Can you work these out from the drawing? Everything is in mm from the part's minimum corner. A direction names the side the tool comes from. Coordinates: 2 decimals unless noted, no trailing zeros. Loops run counter-clockwise (first coordinate to the right, second up) from the corner with the lowest first, then second, coordinate; pieces in that order, holes last. Notation, with made-up numbers: (-22.75, -15) -> (-10.75, -15) arc R24 cw to (-10.75, 22) -> close; hole circle Ø11 at (-4, -19.5). An arc over 180 degrees is marked (long way). Use one line per item in the form item = value. Start each with the question number.
(1) On a 3-axis mill with a long thin cutter (end or side, diameter ignored), from which of +Z, -Z, +X, -X, +Y, -Y can I reach the whole of each face in a straight line? I mean the marked faces 1, 2 and 3. Say none if no direction works.
(2) Thinking about a two-plate mould opening in X: for the marked faces 4, 5, 6 and 7, which applies, released by +X, released by -X, zero draft, split by the parting line, or undercut?
(3) I need wall thicknesses on line 1 (Y direction, x = 1, z = 12.75). Which ranges of the line are inside material? Lowest first, please. Write a range as [from, to].
(4) Imagine slicing it at A-A (x = 6.5). List the corners of the cut face in (y, z) for me, plus the area to 3 significant figures.
(5) I'm going to push a flat-ended pin straight in: pin 1 (0.6 mm diameter, centred on x = 7.5, y = 14, fed in from -Z). Where does the tip first touch, or does it pass through?
(6) Imagine slicing it at B-B (z = 13.5). List the corners of the cut face in (x, y) for me, plus the area to 3 significant figures.
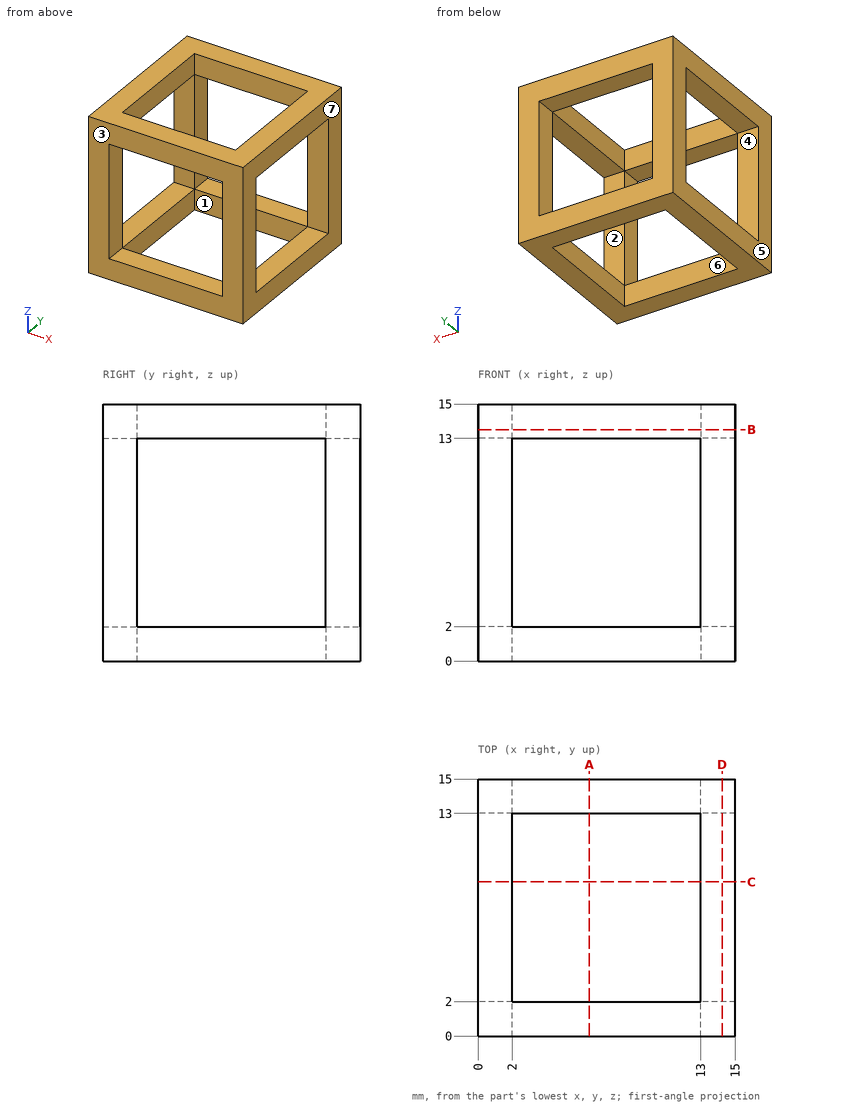
Worked out:
q1.face_1 = +Z, -Z
q1.face_2 = +X, -X
q1.face_3 = +Z, -Z, +X, -X, -Y
q2.face_4 = zero draft
q2.face_5 = released by -X
q2.face_6 = undercut
q2.face_7 = released by +X
q3.line_1 = [0, 2], [13, 15]
q4.outline = (0, 0) -> (2, 0) -> (2, 2) -> (0, 2) -> close; (0, 13) -> (2, 13) -> (2, 15) -> (0, 15) -> close; (13, 0) -> (15, 0) -> (15, 2) -> (13, 2) -> close; (13, 13) -> (15, 13) -> (15, 15) -> (13, 15) -> close
q4.area = 16.0 mm2
q5.pin_1 = 0
q6.outline = (0, 0) -> (15, 0) -> (15, 15) -> (0, 15) -> close; hole (2, 2) -> (13, 2) -> (13, 13) -> (2, 13) -> close
q6.area = 104 mm2
